Verification items for this drawing (mm, ordinates from the low corner). Coordinates: 2 decimals unless noted, no trailing zeros. Order: outer loops, then holes, each group sorted by start corner. A loop starts at its lowest first (then second) coordinate and runs counter-clockwise, first axis right, second up. Notation, with made-up numbers: M 18,68.25 L 27,68.25 A10 ccw 27,72.25 Z; hole C 39.5,29.5 d5. An arc over 180 degrees is marked long. Return JSON: item names as keys, results as strings. Group by question number.
1. Section check B-B, the plane y = 3.5. Record the cut outline in (x, z) (1 decimal).
2. Mould release check, pull along X, two halves, no side actions. Record for the marked faces 1 and 2: +X half, -X half, draft (parallel to the pull), parting line (faces both ways), or undercut.
3. Gauge pin test, flat ends, axial feed: pin 1 (10 mm diameter, centred on x = 129, z = 20.5, fed in from -Y); pin 2 (5 mm diameter, centred on x = 63.5, y = 16, fed in from -Z); pin 3 (1 mm diameter, centred on x = 67.5, y = 20, fed in from +Z) (3 decimals); pin 4 (10 mm diameter, centred on y = 21, z = 6.5, fed in from -X). Record the tip position at first contact, or that the pin passes through.
4. Material ranges on line 1 along Y through (x, z) = (29, 31); line 2 along X through (y, z) = (19, 42.5) (1 decimal); line 3 along Z through (x, y) = (20.5, 14.5), recorded low to high.
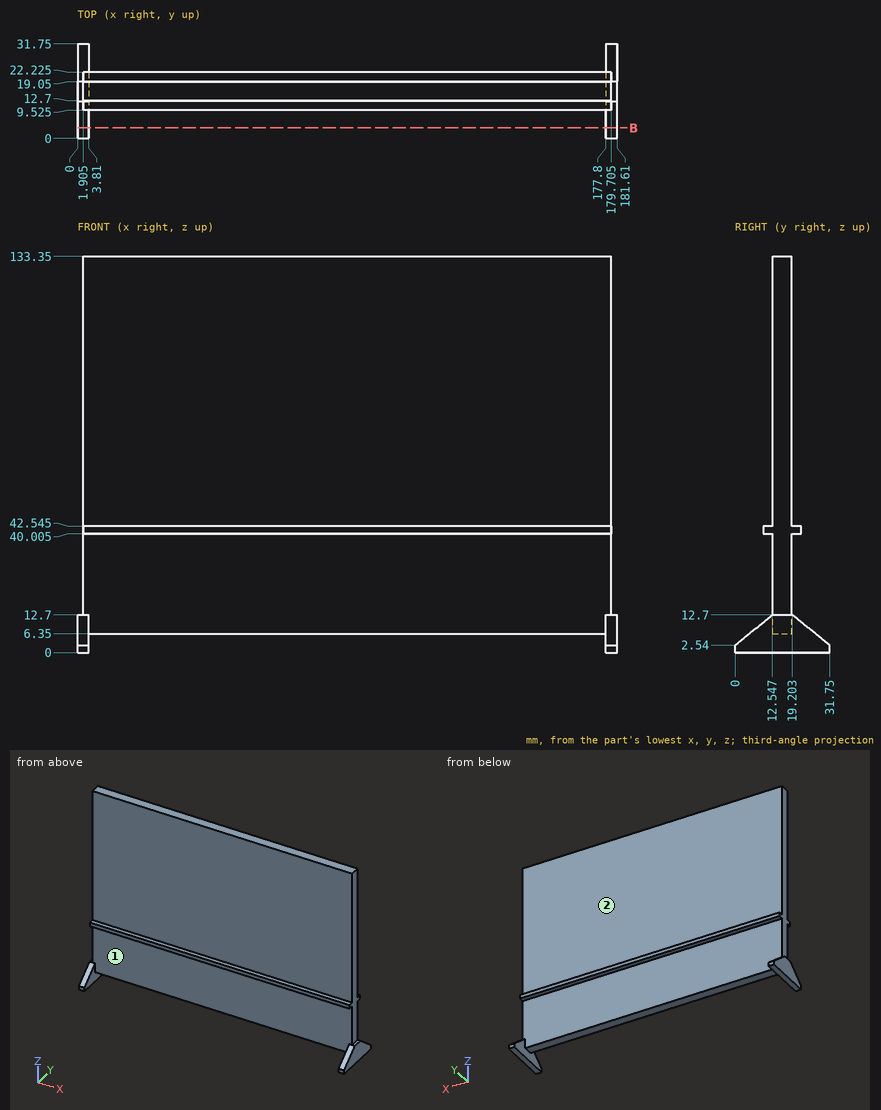
Answers follow:
{
 "1": {"outline": "M 0,0 L 3.8,0 L 3.8,5.4 L 0,5.4 Z; M 177.8,0 L 181.6,0 L 181.6,5.4 L 177.8,5.4 Z"},
 "2": {"face 1": "undercut", "face 2": "draft"},
 "3": {"pin 1": "y = 12.7", "pin 2": "z = 6.35", "pin 3": "z = 42.545", "pin 4": "x = 0"},
 "4": {"line 1": "12.7 to 19.05", "line 2": "1.9 to 179.7", "line 3": "6.35 to 133.35"}
}
